Autodesk Inventor part; units mm, degrees
ref_plane "Work Plane1" through (-10, 0, 28) normal (0, -1, 0) x (1, 0, 0)
ref_plane "YZ Plane" through (0, 0, 0) normal (1, 0, 0) x (0, 1, 0)
ref_plane "XZ Plane" through (0, 0, 0) normal (0, 1, 0) x (-1, 0, 0)
ref_plane "Work Plane1" through (-10, 0, 28) normal (0, -1, 0) x (1, 0, 0)
sketch "Sketch3" plane through (-10, 0, 28) normal (0, -1, 0) x (1, 0, 0)
  line L0 (-10, -28) -> (10, -28)
  line L1 (10, -28) -> (10, 28)
  line L2 (10, 28) -> (-10, 28)
  line L3 (-10, 28) -> (-10, -28)
  line L4 (10, 28) -> (-10, 28)
  line L5 (-10, 28) -> (-10, 31)
  line L6 (-10, 31) -> (10, 31)
  line L7 (10, 31) -> (10, 28)
  line L8 (10, -28) -> (-10, -28)
  line L9 (-10, -28) -> (-10, -31)
  line L10 (-10, -31) -> (10, -31)
  line L11 (10, -31) -> (10, -28)
  line L12 (10, 28) -> (5, 28)
  line L13 (5, 28) -> (5, -28)
  line L14 (-10, 28) -> (-5, 28)
  line L15 (-5, 28) -> (-5, -28)
  line L16 (5, 28) -> (5, 14)
  circle A0 centre (5, 14) radius 1.5
  line L17 (5, 14) -> (5, 4)
  circle A1 centre (5, 4) radius 1.5
  line L18 (10, 28) -> (10, 0)
  line L19 (10, 0) -> (-10, 0)
  circle A2 centre (0, 0) radius 3
  line L20 (0, 28) -> (0, -28)
  circle A3 centre (-5, 4) radius 1.5
  circle A4 centre (-5, 14) radius 1.5
  circle A5 centre (5, -14) radius 1.5
  circle A6 centre (5, -4) radius 1.5
  circle A7 centre (-5, -4) radius 1.5
  circle A8 centre (-5, -14) radius 1.5
  point P0 (10, -28)
  point P1 (-10, 28)
  dimension "d13" = 20
  dimension "d14" = 56
  dimension "d15" = 3
  dimension "d16" = 3
  dimension "d17" = 5
  dimension "d18" = 5
  dimension "d19" = 14
  dimension "d20" = 3
  dimension "d21" = 10
  dimension "d22" = 3
  dimension "d23" = 6
extrude "Extrusion2" add sketch "Sketch3" along normal blind 2 contours L3 L19 L15 A7 A8 L0 | L15 A8 A7 L19 A2 L20 L0 | L3 L2 L15 A4 A3 L19 | L20 A2 L19 L13 A6 A5 L0 | A8 L15 | L15 A8 | L15 A3 A4 L2 L20 A2 L19 | L13 A5 A6 L19 L1 L0 | L20 L19 A2 | A2 L19 L20 | A3 L15 | L15 A3 | A7 L15 | L15 A7 | A2 L20 L19 | A5 L13 | L13 A5 | A2 L20 L2 L13 A0 A1 L19 | L19 L20 A2 | A4 L15 | L15 A4 | L19 L13 A1 A0 L2 L1 | A6 L13 | L13 A6 | A1 L13 | L13 A1 | A0 L13 | L13 A0
sketch "Sketch5" plane through (-10, 0, 28) normal (0, 1, 0) x (1, 0, 0)
  line L0 (-10, -28) -> (-10, 28)
  line L1 (10, 28) -> (-10, 28)
  line L2 (-10, 28) -> (-10, 26)
  line L3 (-10, 26) -> (10, 26)
  line L4 (10, 26) -> (10, 28)
  line L5 (10, 28) -> (10, -28)
  line L6 (10, -28) -> (-10, -28)
  line L7 (-10, -28) -> (-10, -26)
  line L8 (-10, -26) -> (10, -26)
  line L9 (10, -26) -> (10, -28)
  dimension "d26" = 2
  dimension "d27" = 2
extrude "Extrusion3" add sketch "Sketch5" along normal blind 20 contours L0 L1 L4 L3
sketch "Sketch6" plane through (0, -2, 0) normal (0, 0, -1) x (-1, 0, 0)
  line L0 (0, 22) -> (20, 22)
  circle A0 centre (10, 22) radius 10
  point P0 (0, 2)
extrude "Extrusion4" add sketch "Sketch6" against normal up to surface (2 mm away) contours A0 L0 picked at (13.2365, 22.7977)
sketch "Sketch7" plane through (0, -2, 0) normal (0, 0, -1) x (-1, 0, 0)
  arc A0 (20, 22) -> (0, 22) centre (10, 22) ccw
  circle A1 centre (10, 22) radius 7
  circle A2 centre (10, 15) radius 1.5
  circle A3 centre (3, 22) radius 1.5
  circle A4 centre (10, 29) radius 1.5
  circle A5 centre (17, 22) radius 1.5
  point P0 (0, 2)
  dimension "d32" = 14
  dimension "d33" = 3
  dimension "d34" = 3
  dimension "d35" = 3
  dimension "d36" = 3
extrude "Extrusion5" cut sketch "Sketch7" against normal blind 10 contours A1 A5 | A1 A5 | A4 A1 | A1 A4 | A2 A1 | A1 A2 | A3 A1 | A1 A3
ref_plane "Work Plane2" through (-20, 0, 28) normal (0, 0, 1) x (1, 0, 0)
mirror "Mirror1" about plane through (-20, 0, 28) normal (0, 0, 1) of "Extrusion4", "Extrusion5", "Extrusion3"
properties part number "Bracket"
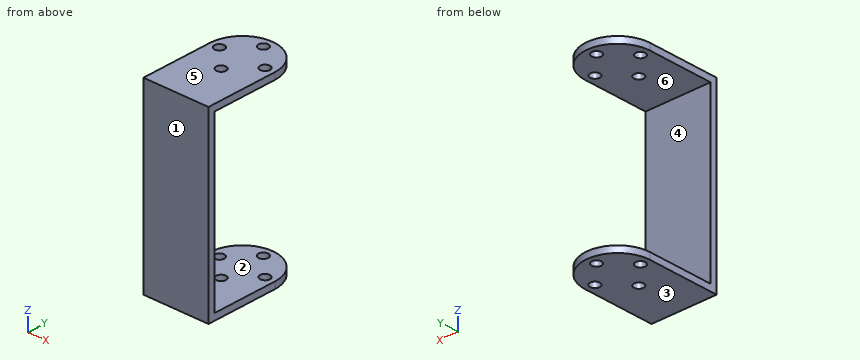
The listing builds one solid part. Answer for the finished solid, in the listing's coordinates (mm). Face numbers are marked on the shaded views. A direction names the side the tool comes from. Round coordinates to 2 decimals unless told otherwise and drop trailing zeros. Order: outer loops, then holes, each group sorted by start corner. A loop starts at its lowest first (then second) coordinate and runs counter-clockwise, first axis right, second up. Notation, with made-up numbers: (37, 3.25) -> (84, 3.25) arc R5 cw to (84, 9.25) -> close; hole circle Ø3 at (-4.5, -37.5). An arc over 180 degrees is marked (long way). Put each result on its own line as item: value.
Q1. Section C-C, the plane x = -10 is taken. Write down the section's boundary in (y, z).
Results list:
outline: (-2, 0) -> (11.5, 0) -> (11.5, 2) -> (0, 2) -> (0, 54) -> (11.5, 54) -> (11.5, 56) -> (-2, 56) -> close; (14.5, 0) -> (25.5, 0) -> (25.5, 2) -> (14.5, 2) -> close; (14.5, 54) -> (25.5, 54) -> (25.5, 56) -> (14.5, 56) -> close; (28.5, 0) -> (30, 0) -> (30, 2) -> (28.5, 2) -> close; (28.5, 54) -> (30, 54) -> (30, 56) -> (28.5, 56) -> close
Q2. Section B-B, the plane y = 13 is taken. Write down the section's boundary in (x, z), and give its area (3 significant figures).
Results list:
outline: (-20, 0) -> (-11.5, 0) -> (-11.5, 2) -> (-20, 2) -> close; (-20, 54) -> (-11.5, 54) -> (-11.5, 56) -> (-20, 56) -> close; (-8.5, 0) -> (0, 0) -> (0, 2) -> (-8.5, 2) -> close; (-8.5, 54) -> (0, 54) -> (0, 56) -> (-8.5, 56) -> close
area: 68.0 mm^2
Q3. This flat-tipped pin is pushed along its axis until it touches: P1, Ø2, axis at x = -10.5, z = 19.5, coming from the +Y side. Where does it stop, or does it pass through?
Results list:
P1: y = 0
Q4. Section D-D, the plane x = -3 is taken. Write down the section's boundary in (y, z).
Results list:
outline: (-2, 0) -> (18.5, 0) -> (18.5, 2) -> (0, 2) -> (0, 54) -> (18.5, 54) -> (18.5, 56) -> (-2, 56) -> close; (21.5, 0) -> (27.14, 0) -> (27.14, 2) -> (21.5, 2) -> close; (21.5, 54) -> (27.14, 54) -> (27.14, 56) -> (21.5, 56) -> close
Q5. Determine the mould class of the marked faces 3, 4, 5 and 6 for opening direction Z: pulls with the +Z half, pulls with the -Z half, needs draft (parallel to the pull), parting line crosses it, or undercut.
Results list:
face 3: pulls with the -Z half
face 4: undercut
face 5: pulls with the +Z half
face 6: undercut
Q6. Which of the six approach directions +Z, -Z, +X, -X, +Y, -Y give full straight-line access (tool end or side, diameter ignored) to the marked faces 1 and 2?
Results list:
face 1: +Z, -Z, +X, -X, -Y
face 2: +X, -X, +Y
Q7. Section A-A, the plane y = 17 is taken. Write down the section's boundary in (x, z), and give its area (3 significant figures).
Results list:
outline: (-20, 0) -> (0, 0) -> (0, 2) -> (-20, 2) -> close; (-20, 54) -> (0, 54) -> (0, 56) -> (-20, 56) -> close
area: 80.0 mm^2
Q8. Consider line 1 along Z through (x, y) = (-5.5, 22); line 2 along X through (y, z) = (20, 54.7); line 3 along X through (y, z) = (13, 0.9). Determine where each line is inside the solid, lowest interval first.
Results list:
line 1: 0 to 2, 54 to 56
line 2: -20 to -18.5, -15.5 to -4.5, -1.5 to 0
line 3: -20 to -11.5, -8.5 to 0
